```python
from build123d import *

# Parameters (mm, degrees)
SKETCH1_R           = 4.7625
BOSS_EXTRUDE1_DEPTH = 19.05
SKETCH2_W           = 9.525
SKETCH2_H           = 1.905
CUT_EXTRUDE1_DEPTH  = 3.175
SKETCH3_R           = 2
CUT_EXTRUDE2_DEPTH  = 8


with BuildPart() as part:
    # Sketch1 → Boss-Extrude1 (new body)
    with BuildSketch(Plane(origin=(0, 0, 0), x_dir=(1, 0, 0), z_dir=(0, 1, 0))):
        Circle(SKETCH1_R)
    extrude(amount=-BOSS_EXTRUDE1_DEPTH)

    # Sketch2 → Cut-Extrude1 (cut)
    with BuildSketch(Plane(origin=(0, 0, 0), x_dir=(1, 0, 0), z_dir=(0, 1, 0))):
        Rectangle(SKETCH2_W, SKETCH2_H)
    extrude(amount=-CUT_EXTRUDE1_DEPTH, mode=Mode.SUBTRACT)

    # Sketch3 → Cut-Extrude2 (cut)
    with BuildSketch(Plane.XZ.offset(19.05)):
        Circle(SKETCH3_R)
    extrude(amount=-CUT_EXTRUDE2_DEPTH, mode=Mode.SUBTRACT)


solid = part.part
```
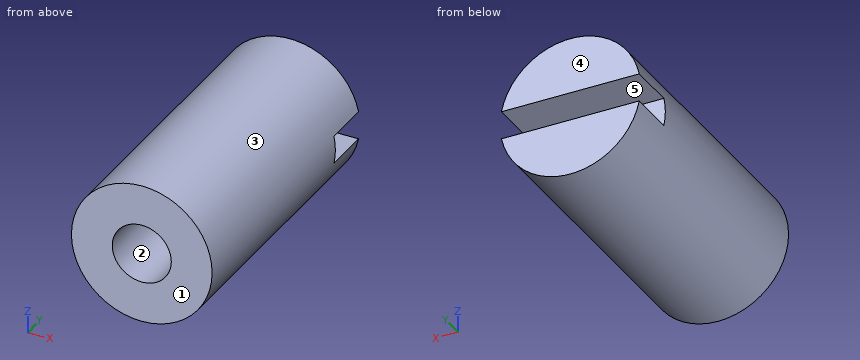
Input: part model. Units: mm. Frame: model coordinates. Face numbers are marked on the shaded views. A direction names the side the tool comes from. Give positions to 0.01 mm unless a question says otherwise; leave off trailing zeros. Order: outer loops, then holes, each group sorted by start corner. A loop starts at its lowest first (then second) coordinate and runs counter-clockwise, first axis right, second up. Notation, with made-up numbers: (72.5, 52.5) -> (82.5, 52.5) arc R18 ccw to (82.5, 75.5) -> close; hole circle Ø7 at (20.5, -34). An arc over 180 degrees is marked (long way). Write each question's results on one line, items separated by ' | '. Start each with the question number.
Item 1: Cut plane D-D on y = -11.75. Return the cut outline in (x, z) (1 decimal).
Item 2: Line query: line 1 (Z direction, x = 0, y = -16.25); line 2 (Y direction, x = 2.25, z = 0.5) (3 decimals); line 3 (Y direction, x = 1.25, z = -1). Output: solid intervals per line, ascending.
Item 3: Mould query, pull axis Z, two halves, no side actions, for the marked faces 1, 2 and 3. Classes: pulls with the +Z half, pulls with the -Z half, needs draft (parallel to the pull), parting line crosses it, or undercut.
Item 4: Cut plane A-A on y = -1.75. Return the cut outline in (x, z) (1 decimal).
Item 5: Contact query for flat-ended pins moving along their axis: P1, Ø3, axis at x = -0.5, z = 1, coming from the -Y side; P2, Ø1, axis at y = -14.5, z = 2.5, coming from the +X side; P3, Ø2.5, axis at x = 1.5, y = -1, coming from the -Z side; P4, Ø1, axis at x = 0.5, z = 0, coming from the +Y side (3 decimals). Output: stop coordinate, or through.
Item 6: Set-up query: the marked faces 4 and 5. Return all of +Z, -Z, +X, -X, +Y, -Y with unobstructed straight access to the full face (end or side cutting, diameter ignored); none if empty.
Established:
1) outline: circle Ø9.5 at (0, 0); hole circle Ø4 at (0, 0)
2) line 1: -4.76 to -2, 2 to 4.76 | line 2: -19.05 to -3.175 | line 3: -11.05 to 0
3) face 1: needs draft | face 2: undercut | face 3: parting line crosses it
4) outline: (-4.7, -1) arc R4.8 ccw to (4.7, -1) -> close; (-4.7, 1) -> (4.7, 1) arc R4.8 ccw to start
5) P1: y = -19.05 | P2: x = 4.32 | P3: z = -4.76 | P4: y = -3.175
6) face 4: +Z, -Z, +X, -X, +Y | face 5: +X, -X, +Y
